from build123d import *

# Parameters (mm, degrees)
F1_DEPTH  = 1160
F2_T      = -1.5
F3_W      = 1157
F3_H      = 1.5
F4_DEPTH  = 180
F5_W      = 1157
F5_H      = 1.5
F6_DEPTH  = 35
F7_W      = 1157
F7_H      = 1.5
F8_DEPTH  = 170
F9_W      = 1160
F9_H      = 80
F10_DEPTH = 1.5
F11_R     = 65
F11_R_2   = 40
F11_W     = 250
F11_H     = 138
F12_DEPTH = 1.5
F14_DEPTH = 245.001
F15_R     = 2.5
F16_DEPTH = 1160.001


with BuildPart() as f1:
    # F0 (on Right) → F1 (new body)
    with BuildSketch(Plane.YZ):
        Polygon((0, 30), (0, 0), (310, 0), (310, 280), (130, 280), align=None)
    extrude(amount=F1_DEPTH)

    # F2
    f2_openings = [f1.faces().sort_by_distance(p)[0] for p in [
        (580, 65, 155),
        (580, 220, 280),
        (580, 0, 15),
        (580, 155, 0),
    ]]
    offset(amount=F2_T, openings=f2_openings)

    # F3 (on face) → F4 (join)
    with BuildSketch(Plane.XZ.offset(-308.5)):
        with Locations((580, 279.25)):
            Rectangle(F3_W, F3_H)
    extrude(amount=F4_DEPTH)

    # F5 (on face) → F6 (join)
    with BuildSketch(Plane(origin=(0, 0, 278.5), x_dir=(1, 0, 0), z_dir=(0, 0, -1))):
        with Locations((580, -129.25)):
            Rectangle(F5_W, F5_H)
    extrude(amount=F6_DEPTH)

    # F7 (on face) → F8 (join)
    with BuildSketch(Plane(origin=(0, 130, 0), x_dir=(-1, 0, 0), z_dir=(0, 1, 0))):
        with Locations((-580, 244.25)):
            Rectangle(F7_W, F7_H)
    extrude(amount=F8_DEPTH)

    # F9 (on face) → F10 (cut)
    with BuildSketch(Plane(origin=(0, 310, 0), x_dir=(-1, 0, 0), z_dir=(0, 1, 0))):
        with Locations((-580, 40)):
            Rectangle(F9_W, F9_H)
    extrude(amount=-F10_DEPTH, mode=Mode.SUBTRACT)

    # F11 (on face) → F12 (cut, through all)
    with BuildSketch(Plane.XY.offset(280)):
        with Locations((85, 219.25)):
            Circle(F11_R)
        with Locations((235, 219.25)):
            Circle(F11_R)
        with Locations((385, 219.25)):
            Circle(F11_R)
        with Locations((535, 174.25)):
            Circle(F11_R_2)
        with Locations((625, 174.25)):
            Circle(F11_R_2)
        with Locations((715, 174.25)):
            Circle(F11_R_2)
        with BuildLine():
            ThreePointArc((513.767183, 256.805709), (512.01903, 241.26903), (527.555709, 243.017183))
            ThreePointArc((527.555709, 243.017183), (550.909903, 248.340097), (556.232817, 271.694291))
            ThreePointArc((556.232817, 271.694291), (557.98097, 287.23097), (542.444291, 285.482817))
            ThreePointArc((542.444291, 285.482817), (519.090097, 280.159903), (513.767183, 256.805709))
        make_face()
        with BuildLine():
            ThreePointArc((616.232817, 271.694291), (617.98097, 287.23097), (602.444291, 285.482817))
            ThreePointArc((602.444291, 285.482817), (579.090097, 280.159903), (573.767183, 256.805709))
            ThreePointArc((573.767183, 256.805709), (572.01903, 241.26903), (587.555709, 243.017183))
            ThreePointArc((587.555709, 243.017183), (610.909903, 248.340097), (616.232817, 271.694291))
        make_face()
        with BuildLine():
            ThreePointArc((676.232817, 271.694291), (677.98097, 287.23097), (662.444291, 285.482817))
            ThreePointArc((662.444291, 285.482817), (639.090097, 280.159903), (633.767183, 256.805709))
            ThreePointArc((633.767183, 256.805709), (632.01903, 241.26903), (647.555709, 243.017183))
            ThreePointArc((647.555709, 243.017183), (670.909903, 248.340097), (676.232817, 271.694291))
        make_face()
        with BuildLine():
            ThreePointArc((736.232817, 271.694291), (737.98097, 287.23097), (722.444291, 285.482817))
            ThreePointArc((722.444291, 285.482817), (699.090097, 280.159903), (693.767183, 256.805709))
            ThreePointArc((693.767183, 256.805709), (692.01903, 241.26903), (707.555709, 243.017183))
            ThreePointArc((707.555709, 243.017183), (730.909903, 248.340097), (736.232817, 271.694291))
        make_face()
        with Locations((975, 219.25)):
            Rectangle(F11_W, F11_H)
    extrude(amount=-F12_DEPTH, mode=Mode.SUBTRACT)

    # F13 (on face) → F14 (cut, through all)
    with BuildSketch(Plane.XY.offset(245)):
        with BuildLine():
            Line((765, 300), (490, 300))
            Line((490, 300), (490, 240))
            ThreePointArc((490, 240), (492.928932, 232.928932), (500, 230))
            Line((500, 230), (755, 230))
            ThreePointArc((755, 230), (762.071068, 232.928932), (765, 240))
            Line((765, 240), (765, 300))
        make_face()
    extrude(amount=-F14_DEPTH, mode=Mode.SUBTRACT)

    # F15 (on face) → F16 (cut, through all)
    with BuildSketch(Plane.YZ.offset(1160)):
        with Locations((260, 15)):
            Circle(F15_R)
        with Locations((50, 15)):
            Circle(F15_R)
    extrude(amount=-F16_DEPTH, mode=Mode.SUBTRACT)


solid = f1.part
For this review, take the finished solid that the model builds, in its own axes (mm). A direction names the side the tool comes from. Coordinates: 2 decimals unless noted, no trailing zeros. Loops run counter-clockwise (first coordinate to the right, second up) from the corner with the lowest first, then second, coordinate; pieces in that order, holes last. Notation, with made-up numbers: (88.5, -24.75) -> (93.5, -24.75) arc R14 ccw to (93.5, -3.75) -> close; hole circle Ø11 at (70.5, -9.75). An arc over 180 degrees is marked (long way). Write each question's results on one line, items separated by ' | '.
Q1. For pin 1 Ø0.8 at (x, y) = (531.5, 309.5) entering from -Z; pin 2 Ø1.6 at (x, z) = (1159, 28.5) entering from +Y; pin 3 Ø6 at (x, y) = (342, 127) entering from -Z, all flat-tipped, find the tip position at first contact; note any pin that passes through.
Taken from the geometry:
pin 1: z = 80 | pin 2: y = 308.5 | pin 3: z = 243.5
Q2. Add section D-D, the plane x = 932.5. State the section outline as (y, z) points, then the cut area to 4 significant figures.
Taken from the geometry:
outline: (128.5, 243.5) -> (300, 243.5) -> (300, 245) -> (130, 245) -> (130, 278.5) -> (150.25, 278.5) -> (150.25, 280) -> (128.5, 280) -> close; (288.25, 278.5) -> (308.5, 278.5) -> (308.5, 80) -> (310, 80) -> (310, 280) -> (288.25, 280) -> close | area: 670.5 mm²
Q3. To check wall thickness, follow line 1 along X through (y, z) = (108.5, 101.5); line 2 along Y through (x, z) = (939.5, 249); line 3 along Z through (x, y) = (103.5, 151.5). State the ranges of each line that lie inside material, in increasing order. Write a range as [from, to].
Taken from the geometry:
line 1: [0, 1.5], [1158.5, 1160] | line 2: [128.5, 130], [308.5, 310] | line 3: [243.5, 245], [278.5, 280]
Q4. Mouldability with a two-part tool opening along Z and no side actions: class faces 4 (the flat face through (588, 213, 243.5)), 5 (the flat face through (572, 308.5, 178)), 6 (the flat face through (572, 130, 262)) as +Z half, -Z half, draft (parallel to the pull), parting line (faces both ways), or undercut.
Taken from the geometry:
face 4: -Z half | face 5: draft | face 6: undercut
Q5. Add section B-B, the plane x = 385. State the section outline as (y, z) points.
Taken from the geometry:
outline: (128.5, 243.5) -> (300, 243.5) -> (300, 245) -> (130, 245) -> (130, 278.5) -> (154.25, 278.5) -> (154.25, 280) -> (128.5, 280) -> close; (284.25, 278.5) -> (308.5, 278.5) -> (308.5, 80) -> (310, 80) -> (310, 280) -> (284.25, 280) -> close
Q6. Machinability: for faces 1 (the flat face through (572, 220, 278.5)), 2 (the cylindrical face through (519.342, 280.408, 279.26)), 3 (the cylindrical face through (445.04, 194.35, 279.26)), which of the approach directions +Z, -Z, +X, -X, +Y, -Y give a long, thin tool a straight path to every point of the face, cutting with its end or side? Answer none if there is none.
Taken from the geometry:
face 1: none | face 2: +Z, -Z | face 3: +Z
Q7. Add section C-C, the plane z = 183. State the section outline as (x, y) points, then the cut area to 3 significant figures.
Taken from the geometry:
outline: (0, 79.56) -> (1.5, 79.56) -> (1.5, 308.5) -> (1158.5, 308.5) -> (1158.5, 79.56) -> (1160, 79.56) -> (1160, 310) -> (0, 310) -> close | area: 2,430 mm²
Q8. Add section A-A, the plane y = 71.5. State the section outline as (x, z) points.
Taken from the geometry:
outline: (0, 0) -> (1.5, 0) -> (1.5, 167.5) -> (0, 167.5) -> close; (1158.5, 0) -> (1160, 0) -> (1160, 167.5) -> (1158.5, 167.5) -> close
